For this review, take the finished solid that the model builds, in its own axes (mm). A direction names the side the tool comes from. Give positions to 0.01 mm unless a question says otherwise; leave off trailing zeros. Write each loop counter-clockwise with the first axis right and the second up, starting at its lowest first coordinate (ties: lowest second). Pieces come first, ordered by that corner, then holes. Notation, with made-up numbers: (42.25, 30) -> (95.25, 30) arc R21 ccw to (95.25, 59) -> close; hole circle Ø8 at (36, 49.25). An arc over 180 degrees is marked (long way). Return JSON: item names as keys, results as strings.
from build123d import *

# Parameters (mm, degrees)
BOSS_EXTRUDE1_DEPTH = 1.5875
SKETCH2_W           = 3.3782
SKETCH2_H           = 6.477
SKETCH2_H_2         = 12.7
CUT_EXTRUDE1_DEPTH  = 4.175


with BuildPart() as part:
    # Sketch1 → Boss-Extrude1 (new body, symmetric)
    with BuildSketch(Plane.XY):
        with BuildLine():
            Line((0, -97.563004684), (0, -84.863004684))
            ThreePointArc((0, -84.863004684), (45.091480007, -102.953300884), (92.3925, -114.048970912))
            ThreePointArc((92.3925, -114.048970912), (339.042339878, -117.088496575), (583.522463964, -84.303573898))
            Line((583.522463964, -84.303573898), (583.522463964, -97.003573898))
            ThreePointArc((583.522463964, -97.003573898), (339.198389145, -132.023125314), (92.3925, -129.288970912))
            ThreePointArc((92.3925, -129.288970912), (44.158404147, -119.360611557), (0, -97.563004684))
        make_face()
    extrude(amount=BOSS_EXTRUDE1_DEPTH, both=True)

    # Sketch2 → Cut-Extrude1 (cut, through all)
    with BuildSketch(Plane.XY.offset(1.5875)):
        with Locations((1.6891, -88.101504684)):
            Rectangle(SKETCH2_W, SKETCH2_H)
        with Locations((93.98, -114.06579143)):
            Rectangle(SKETCH2_W, SKETCH2_H_2)
        Polygon((191.155368795, -126.195526401), (194.532828758, -126.124819669), (194.267013976, -113.427601765), (190.889554014, -113.498308497), align=None)
    extrude(amount=-CUT_EXTRUDE1_DEPTH, mode=Mode.SUBTRACT)


solid = part.part
1. To check wall thickness, follow probe 1 along Y at (x, z) = (222, 0.2); probe 2 along Y at (x, z) = (533, 0). State the ranges of each line that lie inside material, in increasing order.
Results found:
{"probe 1": "y = -135.45 to -120.13", "probe 2": "y = -107.41 to -94.07"}
2. The part is to be moulded in two halves that separate along X. For faces 3 (the flat face through (293, -121, 1.588)), 4 (the cylindrical face through (387.25, -113.48, 0.02)), 5 (the cylindrical face through (44.813, -119.584, 0.022)), say which applies: +X half, -X half, draft (parallel to the pull), parting line (faces both ways), or undercut.
Results found:
{"face 3": "draft", "face 4": "undercut", "face 5": "-X half"}
3. Add section C-C, the plane x = 208. State the section outline as (y, z) points, plus the area to 3 significant figures.
Results found:
{"outline": "(-135.29, -1.59) -> (-119.95, -1.59) -> (-119.95, 1.59) -> (-135.29, 1.59) -> close", "area": "48.7 mm²"}
4. Add section B-B, the plane y = -102.5. State the section outline as (x, z) points.
Results found:
{"outline": "(7.83, -1.59) -> (43.67, -1.59) -> (43.67, 1.59) -> (7.83, 1.59) -> close; (480.82, -1.59) -> (557.85, -1.59) -> (557.85, 1.59) -> (480.82, 1.59) -> close"}
5. For faces 1 (the flat face through (293, -121, -1.588)), 2 (the cylindrical face through (46.2, -103.3, 0)), list the 3-axis set-ups (+Z, -Z, +X, -X, +Y, -Y) from which the entire face can be reached by the end or side of a thin tool; tool diameter is ignored.
Results found:
{"face 1": "-Z, +X, -X, +Y, -Y", "face 2": "+Z, -Z, +Y"}
6. Add section D-D, the plane x = 113.5. State the section outline as (y, z) points.
Results found:
{"outline": "(-131.01, -1.59) -> (-115.72, -1.59) -> (-115.72, 1.59) -> (-131.01, 1.59) -> close"}
7. Add section A-A, the plane z = -1.05. State the section outline as (x, y) points, plus the area to 3 significant figures.
Results found:
{"outline": "(0, -97.56) arc R193.24 ccw to (92.39, -129.29) arc R1610.16 ccw to (583.52, -97) -> (583.52, -84.3) arc R1695.33 cw to (194.4, -119.67) -> (194.53, -126.12) -> (191.16, -126.2) -> (191.02, -119.58) arc R1695.33 cw to (95.67, -114.33) -> (95.67, -120.42) -> (92.29, -120.42) -> (92.29, -114.03) arc R321.8 cw to (3.38, -86.5) -> (3.38, -91.34) -> (0, -91.34) -> close", "area": "8,580 mm²"}
8. For pin 1 (1.6 mm diameter, centred on y = -90, z = 0, fed in from -X); pin 2 (1.6 mm diameter, centred on x = 2, z = 0, fed in from +Y), all flat-tipped, find the tip position at first contact; note any pin that passes through.
Results found:
{"pin 1": "stops at x = 3.38", "pin 2": "stops at y = -91.34"}
